Verification items for the finished model (mm, model axes). Face numbers are marked on the shaded views. A direction names the side the tool comes from. Round coordinates to 2 decimals unless told otherwise and drop trailing zeros. Write each loop counter-clockwise with the first axis right and the second up, starting at its lowest first coordinate (ties: lowest second). Pieces come first, ordered by that corner, then holes. Notation, with made-up numbers: (-39.5, 28.5) - (-3.5, 28.5) arc R20 cw to (-3.5, 33.5) - close; hole circle Ø8 at (-19, -13.5). An arc over 180 degrees is marked (long way). Answer as a JSON object with one key per item and string values.
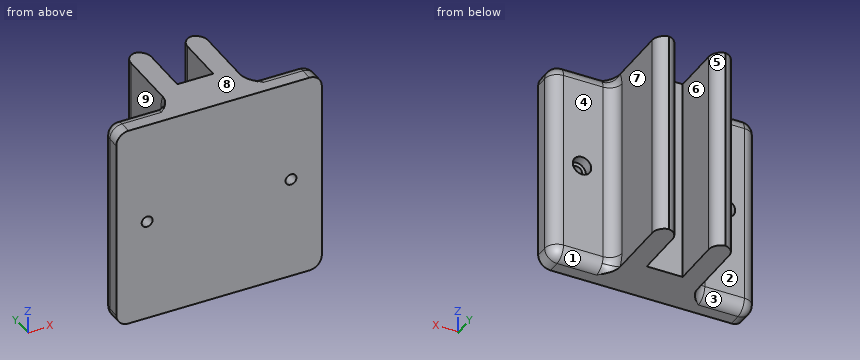
```python
from build123d import *

# Parameters (mm, degrees)
BOSS_EXTRUDE1_DEPTH = 100
SKETCH2_W           = 100
SKETCH2_H           = 100
BOSS_EXTRUDE2_DEPTH = 12
SKETCH3_R           = 4.5
CUT_EXTRUDE1_DEPTH  = 5
SKETCH4_R           = 2.65
CUT_EXTRUDE2_DEPTH  = 7
FILLET1_R           = 6
FILLET3_R           = 6
FILLET4_R           = 6


with BuildPart() as part:
    # Sketch1 → Boss-Extrude1 (new body)
    with BuildSketch(Plane.XY):
        Polygon((0, 0), (-37.5, 0), (-37.5, 40), (-27.5, 40), (-27.5, 10), (-10, 10), (-10, 40), (0, 40), align=None)
    extrude(amount=BOSS_EXTRUDE1_DEPTH)

    # Sketch2 → Boss-Extrude2 (add)
    with BuildSketch(Plane.XZ):
        with Locations((-18.75, 50)):
            Rectangle(SKETCH2_W, SKETCH2_H)
    extrude(amount=BOSS_EXTRUDE2_DEPTH)

    # Sketch3 → Cut-Extrude1 (cut)
    with BuildSketch(Plane(origin=(0, 0, 0), x_dir=(1, 0, 0), z_dir=(0, 1, 0))):
        with Locations(Location((16.25, -50, 0), (0, 0, 180))):
            Circle(SKETCH3_R)
        with Locations(Location((-53.75, -50, 0), (0, 0, 180))):
            Circle(SKETCH3_R)
    extrude(amount=-CUT_EXTRUDE1_DEPTH, mode=Mode.SUBTRACT)

    # Sketch4 → Cut-Extrude2 (cut)
    with BuildSketch(Plane(origin=(0, -5, 0), x_dir=(1, 0, 0), z_dir=(0, 1, 0))):
        with Locations(Location((16.25, -50, 0), (0, 0, 180))):
            Circle(SKETCH4_R)
        with Locations(Location((-53.75, -50, 0), (0, 0, 180))):
            Circle(SKETCH4_R)
    extrude(amount=-CUT_EXTRUDE2_DEPTH, mode=Mode.SUBTRACT)

    # Fillet1
    # the kernel refuses this fillet: 6 mm, written as the material it takes off along each edge
    with BuildSketch(Plane(origin=(25.25, -6, 6), x_dir=(0, 1, 0), z_dir=(1, 0, 0))) as fillet1_piece_1_section:
        Polygon((0, 0), (FILLET1_R, 0), (FILLET1_R, -FILLET1_R), (0, -FILLET1_R), align=None)
    fillet1_piece_1 = extrude(amount=FILLET1_R, mode=Mode.PRIVATE)
    fillet1_piece_1 = fillet1_piece_1 - Plane(origin=(25.25, -6, 6), x_dir=(0, -0.7071067811865475, 0.7071067811865475), z_dir=(1, 0, 0)) * Sphere(FILLET1_R, mode=Mode.PRIVATE)
    add(fillet1_piece_1, mode=Mode.SUBTRACT)
    with BuildSketch(Plane(origin=(25.25, -6, 94), x_dir=(1, 0, 0), z_dir=(0, 0, 1))) as fillet1_piece_2_section:
        Polygon((0, 0), (FILLET1_R, 0), (FILLET1_R, FILLET1_R), (0, FILLET1_R), align=None)
    fillet1_piece_2 = extrude(amount=FILLET1_R, mode=Mode.PRIVATE)
    fillet1_piece_2 = fillet1_piece_2 - Plane(origin=(25.25, -6, 94), x_dir=(-0.7071067811865474, -0.7071067811865477, 0), z_dir=(0, 0, 1)) * Sphere(FILLET1_R, mode=Mode.PRIVATE)
    add(fillet1_piece_2, mode=Mode.SUBTRACT)
    with BuildSketch(Plane(origin=(-62.75, -6, 94), x_dir=(-1, 0, 0), z_dir=(0, 0, 1))) as fillet1_piece_3_section:
        Polygon((0, 0), (FILLET1_R, 0), (FILLET1_R, -FILLET1_R), (0, -FILLET1_R), align=None)
    fillet1_piece_3 = extrude(amount=FILLET1_R, mode=Mode.PRIVATE)
    fillet1_piece_3 = fillet1_piece_3 - Plane(origin=(-62.75, -6, 94), x_dir=(0.7071067811865477, -0.7071067811865474, 0), z_dir=(0, 0, 1)) * Sphere(FILLET1_R, mode=Mode.PRIVATE)
    add(fillet1_piece_3, mode=Mode.SUBTRACT)
    with BuildSketch(Plane(origin=(-62.75, -6, 6), x_dir=(0, 1, 0), z_dir=(-1, 0, 0))) as fillet1_piece_4_section:
        Polygon((0, 0), (FILLET1_R, 0), (FILLET1_R, FILLET1_R), (0, FILLET1_R), align=None)
    fillet1_piece_4 = extrude(amount=FILLET1_R, mode=Mode.PRIVATE)
    fillet1_piece_4 = fillet1_piece_4 - Plane(origin=(-62.75, -6, 6), x_dir=(0, -0.7071067811865475, 0.7071067811865475), z_dir=(-1, 0, 0)) * Sphere(FILLET1_R, mode=Mode.PRIVATE)
    add(fillet1_piece_4, mode=Mode.SUBTRACT)
    with BuildSketch(Plane(origin=(31.25, -6, 0), x_dir=(0, 0, 1), z_dir=(0, -1, 0)), Plane(origin=(31.25, -6, 100), x_dir=(-1, 0, 0), z_dir=(0, -1, 0))) as fillet1_piece_5:
        with BuildLine():
            CenterArc((FILLET1_R, FILLET1_R), FILLET1_R, 180, 90)
            Line((0, FILLET1_R), (0, 0))
            Line((0, 0), (FILLET1_R, 0))
        make_face()
    extrude(amount=21, mode=Mode.SUBTRACT)
    with BuildSketch(Plane(origin=(25.25, 0, 0), x_dir=(0, 0, 1), z_dir=(-1, 0, 0)), Plane(origin=(-37.5, 0, 0), x_dir=(0, 0, 1), z_dir=(-1, 0, 0))) as fillet1_piece_6:
        with BuildLine():
            CenterArc((FILLET1_R, -FILLET1_R), FILLET1_R, 90, 90)
            Line((0, -FILLET1_R), (0, 0))
            Line((0, 0), (FILLET1_R, 0))
        make_face()
    extrude(amount=25.25, mode=Mode.SUBTRACT)
    with BuildSketch(Plane(origin=(31.25, 0, 94), x_dir=(0, -1, 0), z_dir=(0, 0, -1)), Plane(origin=(-68.75, 0, 6), x_dir=(0, -1, 0), z_dir=(0, 0, 1))) as fillet1_piece_7:
        with BuildLine():
            CenterArc((FILLET1_R, FILLET1_R), FILLET1_R, 180, 90)
            Line((0, FILLET1_R), (0, 0))
            Line((0, 0), (FILLET1_R, 0))
        make_face()
    extrude(amount=88, mode=Mode.SUBTRACT)
    with BuildSketch(Plane(origin=(0, 0, 100), x_dir=(0, -1, 0), z_dir=(1, 0, 0)), Plane(origin=(-62.75, 0, 100), x_dir=(0, -1, 0), z_dir=(1, 0, 0))) as fillet1_piece_8:
        with BuildLine():
            CenterArc((FILLET1_R, FILLET1_R), FILLET1_R, 180, 90)
            Line((0, FILLET1_R), (0, 0))
            Line((0, 0), (FILLET1_R, 0))
        make_face()
    extrude(amount=25.25, mode=Mode.SUBTRACT)
    with BuildSketch(Plane(origin=(-68.75, -6, 100), x_dir=(1, 0, 0), z_dir=(0, -1, 0)), Plane(origin=(-68.75, -6, 0), x_dir=(0, 0, 1), z_dir=(0, -1, 0))) as fillet1_piece_9:
        with BuildLine():
            CenterArc((FILLET1_R, -FILLET1_R), FILLET1_R, 90, 90)
            Line((0, -FILLET1_R), (0, 0))
            Line((0, 0), (FILLET1_R, 0))
        make_face()
    extrude(amount=21, mode=Mode.SUBTRACT)
    with BuildSketch(Plane(origin=(-10, 40, -15), x_dir=(1, 0, 0), z_dir=(0, 0, 1)), Plane(origin=(-27.5, 40, -15), x_dir=(0, -1, 0), z_dir=(0, 0, 1)), Plane(origin=(-37.5, 40, -15), x_dir=(1, 0, 0), z_dir=(0, 0, 1)), Plane(origin=(0, 40, -15), x_dir=(0, -1, 0), z_dir=(0, 0, 1))) as fillet1_piece_10:
        with BuildLine():
            CenterArc((FILLET1_R, -FILLET1_R), FILLET1_R, 90, 90)
            Line((0, -FILLET1_R), (0, 0))
            Line((0, 0), (FILLET1_R, 0))
        make_face()
    extrude(amount=130, mode=Mode.SUBTRACT)

    # Fillet3
    fillet3_edges = [part.edges().sort_by_distance(p)[0] for p in [
        (0, 0, 50),
        (0, -1.757359313, 1.757359313),
        (0, -1.757359313, 98.242640687),
    ]]
    fillet(fillet3_edges, radius=FILLET3_R)

    # Fillet4
    # the kernel refuses this fillet: 6 mm, written as the material it adds along each edge
    with BuildSketch(Plane(origin=(-37.5, 0, 6), x_dir=(0, 1, 0), z_dir=(0, 0, 1))) as fillet4_piece_1:
        with BuildLine():
            CenterArc((FILLET4_R, FILLET4_R), FILLET4_R, 180, 90)
            Line((0, FILLET4_R), (0, 0))
            Line((0, 0), (FILLET4_R, 0))
        make_face()
    extrude(amount=88)
    with BuildSketch(Plane(origin=(-37.5, -6, 94), x_dir=(0, 1, 0), z_dir=(0, 0, -1))) as fillet4_piece_2_section:
        with BuildLine():
            CenterArc((6 + FILLET4_R, -FILLET4_R), FILLET4_R, 90, 90)
            Line((6 + FILLET4_R, 0), (6, 0))
            Line((6, 0), (6, -FILLET4_R))
        make_face()
    fillet4_piece_2 = revolve(axis=Axis((-37.5, -6, 94), (1, 0, 0)), revolution_arc=233.296989237, mode=Mode.PRIVATE)
    fillet4_piece_2 = split(fillet4_piece_2, bisect_by=Plane(origin=(-39.369769667, -1.500366283, 100), z_dir=(0, 0, -1)), keep=Keep.TOP, mode=Mode.PRIVATE)
    fillet4_piece_2 = split(fillet4_piece_2, bisect_by=Plane(origin=(-39.369769667, -12, 98.499633777), z_dir=(0, 1, 0)), keep=Keep.TOP, mode=Mode.PRIVATE)
    add(fillet4_piece_2)
    with BuildSketch(Plane(origin=(-37.5, -6, 6), x_dir=(0, 1, 0), z_dir=(0, 0, 1))) as fillet4_piece_3_section:
        with BuildLine():
            CenterArc((6 + FILLET4_R, FILLET4_R), FILLET4_R, 180, 90)
            Line((6, FILLET4_R), (6, 0))
            Line((6, 0), (6 + FILLET4_R, 0))
        make_face()
    fillet4_piece_3 = revolve(axis=Axis((-37.5, -6, 6), (-1, 0, 0)), revolution_arc=233.296989237, mode=Mode.PRIVATE)
    fillet4_piece_3 = split(fillet4_piece_3, bisect_by=Plane(origin=(-38.503801185, -12, 3.658909584), z_dir=(0, 1, 0)), keep=Keep.TOP, mode=Mode.PRIVATE)
    fillet4_piece_3 = split(fillet4_piece_3, bisect_by=Plane(origin=(-38.503801185, 1.318651502, 0), z_dir=(0, 0, 1)), keep=Keep.TOP, mode=Mode.PRIVATE)
    add(fillet4_piece_3)


solid = part.part
```
1. Cross-section at B-B (y = 13). Record the boundary of the cut face in (x, z), plus the area to 3 significant figures.
Completed:
{"outline": "(-37.5, 0) - (-27.5, 0) - (-27.5, 100) - (-37.5, 100) - close; (-10, 0) - (0, 0) - (0, 100) - (-10, 100) - close", "area": "2,000 mm^2"}
2. Cross-section at D-D (z = 10). Record the boundary of the cut face in (x, y), plus the area to 3 significant figures.
Completed:
{"outline": "(-68.75, -12) - (31.25, -12) - (31.25, -6) arc R6 ccw to (25.25, 0) - (6, 0) arc R6 cw to (0, 6) - (0, 34) arc R6 ccw to (-5, 39.92) arc R6 ccw to (-10, 34) - (-10, 10) - (-27.5, 10) - (-27.5, 34) arc R6 ccw to (-32.5, 39.92) arc R6 ccw to (-37.5, 34) - (-37.5, 6) arc R6 cw to (-43.5, 0) - (-62.75, 0) arc R6 ccw to (-68.75, -6) - close", "area": "2,140 mm^2"}
3. Cross-section at C-C (x = 16.25). Record the boundary of the cut face in (y, z), plus the area to 3 significant figures.
Completed:
{"outline": "(-12, 0) - (-6, 0) arc R6 ccw to (0, 6) - (0, 45.5) - (-5, 45.5) - (-5, 47.35) - (-12, 47.35) - close; (-12, 52.65) - (-5, 52.65) - (-5, 54.5) - (0, 54.5) - (0, 94) arc R6 ccw to (-6, 100) - (-12, 100) - close", "area": "1,100 mm^2"}
4. Access from +Z, -Z, +X, -X, +Y, -Y to the whole of each face (thin tool, end or side, straight path). Record for the marked faces 1, 2, 3, 4 and 5.
Completed:
{"face 1": "-Z, +X, +Y", "face 2": "+Z, -Z, -X, +Y", "face 3": "-Z, -X, +Y", "face 4": "+Z, -Z, +X, +Y", "face 5": "+Z, -Z, +Y"}
5. Cross-section at A-A (z = 50). Count the separate pieces of the cut face and the enclosed holes in it, plus the area to 3 significant figures.
Completed:
{"separate pieces": "3", "enclosed holes": "0", "area": "1,980 mm^2"}
6. Material ranges on probe 1 along Z at (x, y) = (16.25, -6.25); probe 2 along X at (y, z) = (26, 54.5); probe 3 along Y at (x, z) = (20, 57.5), recorded low to high. Write a range as from..to.
Completed:
{"probe 1": "z = 0..47.35, 52.65..100", "probe 2": "x = -37.5..-27.5, -10..0", "probe 3": "y = -12..0"}
7. Mould release check, pull along X, two halves, no side actions. Record for the marked faces 6, 7, 8 and 9: released by +X, released by -X, zero draft, split by the parting line, or undercut.
Completed:
{"face 6": "undercut", "face 7": "released by +X", "face 8": "zero draft", "face 9": "released by -X"}
8. Go/stop test with flat-tipped pins: pin 1 (10 mm diameter, centred on x = 18, z = 49, fed in from +Y); pin 2 (12 mm diameter, centred on y = 24, z = 85.5, fed in from -X); pin 3 (5 mm diameter, centred on x = -17.5, z = 59, fed in from +Y). Record where each tip stops, or that it passes through.
Completed:
{"pin 1": "stops at y = 0", "pin 2": "stops at x = -37.5", "pin 3": "stops at y = 10"}
